```python
from build123d import *

# Parameters (mm, degrees)
UPPER_23_W                      = 2.5
UPPER_23_H                      = 1
BOSS_EXTRUDE9_DEPTH             = 20
SKETCH50_W                      = 8
SKETCH50_H                      = 20
BOSS_EXTRUDE10_DEPTH            = 6
TAP_DRILL_FOR_M4X0_7_TAP2_D     = 3.3
TAP_DRILL_FOR_M4X0_7_TAP2_DEPTH = 20
FILLET1_R                       = 3


with BuildPart() as part:
    # upper_23 → Boss-Extrude9 (new body)
    with BuildSketch(Plane(origin=(0, -19, 0), x_dir=(1, 0, 0), z_dir=(0, 1, 0))):
        Polygon((-4, 12), (-4, 9.5), (-3, 9.5), (-1.556624327, 12), align=None)
        Polygon((-3, 9.5), (-4, 9.5), (-4, 8.5), (-1.25, 8.5), (-1.25, 9.5), (-2.5, 9.5), align=None)
        with Locations((0, 9)):
            Rectangle(UPPER_23_W, UPPER_23_H)
        Polygon((4, 8.5), (4, 9.5), (3, 9.5), (2.5, 9.5), (1.25, 9.5), (1.25, 8.5), align=None)
        Polygon((3, 9.5), (4, 9.5), (4, 12), (1.556624327, 12), align=None)
    extrude(amount=BOSS_EXTRUDE9_DEPTH)

    # Sketch50 → Boss-Extrude10 (add)
    with BuildSketch(Plane.XY.offset(-8.5)):
        with Locations((0, -9)):
            Rectangle(SKETCH50_W, SKETCH50_H)
    extrude(amount=BOSS_EXTRUDE10_DEPTH)

    # Tap Drill for M4x0.7 Tap2
    with Locations(Plane(origin=(0, 1, 0), x_dir=(1, 0, 0), z_dir=(0, 1, 0))):
        with Locations((0, 6)):
            Hole(TAP_DRILL_FOR_M4X0_7_TAP2_D / 2, depth=TAP_DRILL_FOR_M4X0_7_TAP2_DEPTH)

    # Fillet1
    fillet1_edges = [part.edges().sort_by_distance(p)[0] for p in [
        (-4, -9, -2.5),
        (4, -9, -2.5),
    ]]
    fillet(fillet1_edges, radius=FILLET1_R)


solid = part.part
```
Geometry check sheet. Reference: the model listing, model coordinates, mm. A direction names the side the tool comes from. Coordinates: 2 decimals unless noted, no trailing zeros. Order: outer loops, then holes, each group sorted by start corner. A loop starts at its lowest first (then second) coordinate and runs counter-clockwise, first axis right, second up. Notation, with made-up numbers: (75, 15) - (110, 15) arc R27 ccw to (110, 32) - close; hole circle Ø6 at (-14, -0.5). An arc over 180 degrees is marked (long way). Answer as a JSON object with one key per item and string values. Group by question number.
Item 1: Tool access check on faces 5 (the face through (-2.29, -9.14, -10.73)), 6 (the face through (-3, -9, -12)). Record the directions out of +Z, -Z, +X, -X, +Y, -Y that give a thin tool (end or side, any length) a straight path to the whole face; none if there is none.
Item 2: Scan lines: probe 1 along X at (y, z) = (-5.25, -6); probe 2 along Z at (x, y) = (0, -9.25); probe 3 along Z at (x, y) = (2.25, -5.75). Record each from-to range of solid material in increasing order.
Item 3: Sectioned sample at B-B, the plane x = 0. Record the cut outline in (y, z).
Item 4: Sectioned sample at A-A, the plane z = -6. Record the cut outline in (x, y).
Item 5: Draft check along Z on faces 1 (the face through (0.4, -9.1, -4.4)), 2 (the face through (2.268, -9.14, -10.768)), 3 (the face through (0, -19, -8)), 4 (the face through (0, -9, -2.5)). Enter one of: +Z half, -Z half, draft (parallel to the pull), parting line (faces both ways), or undercut.
Item 6: Sectioned sample at C-C, the plane y = -16.5. Record the cut outline in (x, z).
Resolved:
{
 "1": {"face 5": "+Y, -Y", "face 6": "-Z, +X, -X, +Y, -Y"},
 "2": {"probe 1": "-4 to -1.65, 1.65 to 4", "probe 2": "-9.5 to -7.65, -4.35 to -2.5", "probe 3": "-12 to -10.8, -9.5 to -2.77"},
 "3": {"outline": "(-19, -9.5) - (1, -9.5) - (1, -7.65) - (-19, -7.65) - close; (-19, -4.35) - (1, -4.35) - (1, -2.5) - (-19, -2.5) - close"},
 "4": {"outline": "(-4, -19) - (-1.65, -19) - (-1.65, 1) - (-4, 1) - close; (1.65, -19) - (4, -19) - (4, 1) - (1.65, 1) - close"},
 "5": {"face 1": "undercut", "face 2": "undercut", "face 3": "draft", "face 4": "+Z half"},
 "6": {"outline": "(-4, -12) - (-1.56, -12) - (-3, -9.5) - (3, -9.5) - (1.56, -12) - (4, -12) - (4, -5.5) arc R3 ccw to (1, -2.5) - (-1, -2.5) arc R3 ccw to (-4, -5.5) - close; hole circle Ø3.3 at (0, -6)"}
}
